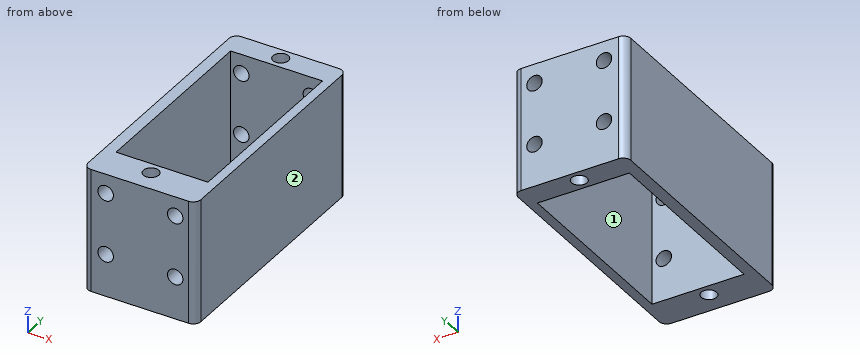
from build123d import *

# Parameters (mm, degrees)
SKETCH2_W           = 14.6
SKETCH2_H           = 32
BOSS_EXTRUDE1_DEPTH = 16
FILLET1_R           = 1
SKETCH3_W           = 11.9
SKETCH3_H           = 24.4
CUT_EXTRUDE1_DEPTH  = 16
SKETCH4_R           = 1
CUT_EXTRUDE2_DEPTH  = 16
SKETCH5_R           = 1
CUT_EXTRUDE3_DEPTH  = 113.555199241


with BuildPart() as part:
    # Sketch2 → Boss-Extrude1 (new body)
    with BuildSketch(Plane.XY):
        with Locations((-99.41772522, 219.327818509)):
            Rectangle(SKETCH2_W, SKETCH2_H)
    extrude(amount=BOSS_EXTRUDE1_DEPTH)

    # Fillet1
    fillet1_edges = [part.edges().sort_by_distance(p)[0] for p in [
        (-106.71772522, 235.327818509, 8),
        (-92.11772522, 235.327818509, 8),
        (-92.11772522, 203.327818509, 8),
        (-106.71772522, 203.327818509, 8),
    ]]
    fillet(fillet1_edges, radius=FILLET1_R)

    # Sketch3 → Cut-Extrude1 (cut)
    with BuildSketch(Plane.XY.offset(16)):
        with Locations((-99.26772522, 219.999996948)):
            Rectangle(SKETCH3_W, SKETCH3_H)
    extrude(amount=-CUT_EXTRUDE1_DEPTH, mode=Mode.SUBTRACT)

    # Sketch4 → Cut-Extrude2 (cut)
    with BuildSketch(Plane.XY.offset(16)):
        with Locations((-99.709122305, 233.799996948)):
            Circle(SKETCH4_R)
        with Locations((-99.709122305, 206.199996948)):
            Circle(SKETCH4_R)
    extrude(amount=-CUT_EXTRUDE2_DEPTH, mode=Mode.SUBTRACT)

    # Sketch5 → Cut-Extrude3 (cut, through all)
    with BuildSketch(Plane(origin=(0, 235.327818509, 0), x_dir=(1, 0, 0), z_dir=(0, 1, 0))):
        with Locations(Location((-103.837557169, -5.5, 0), (0, 0, 270))):
            Circle(SKETCH5_R)
        with Locations(Location((-94.837557169, -5.5, 0), (0, 0, 270))):
            Circle(SKETCH5_R)
        with Locations(Location((-94.837557169, -13.5, 0), (0, 0, 270))):
            Circle(SKETCH5_R)
        with Locations(Location((-103.837557169, -13.5, 0), (0, 0, 270))):
            Circle(SKETCH5_R)
    extrude(amount=-CUT_EXTRUDE3_DEPTH, mode=Mode.SUBTRACT)


solid = part.part
Can you work these out from the model? Positions are in its coordinate system, mm. Face numbers are marked on the shaded views. A direction names the side the tool comes from. Coordinates: 2 decimals unless noted, no trailing zeros. Loops run counter-clockwise (first coordinate to the right, second up) from the corner with the lowest first, then second, coordinate; pieces in that order, holes last. Notation, with made-up numbers: (37.25, 0) - (95.25, 0) arc R31 ccw to (95.25, 35) - close; hole circle Ø5 at (52.25, -1). An arc over 180 degrees is marked (long way). Answer as a JSON object with one key per item and string values. Group by question number.
Item 1: If we section it at A-A (z = 13.5): State how many separate pieces and enclosed holes the cut face has, plus the area to 3 significant figures.
Item 2: On a 3-axis mill with a long thin cutter (end or side, diameter ignored), from which of +Z, -Z, +X, -X, +Y, -Y can I reach the whole of each face in a straight line? I mean the marked faces 1 and 2. Say none if no direction works.
Item 3: If I drill on L1, parallel to X at y = 204.2, z = 5.5; L2, parallel to Y at x = -98.5, z = 8; L3, parallel to X at y = 230.5, z = 14, over which ranges is the centre line in solid material (lowest first)? Write a range as from..to.
Item 4: If we section it at C-C (y = 210.5): List the corners of the cut face in (x, z) for me, plus the area to 3 significant figures.
Item 5: If we section it at B-B (z = 11): List the corners of the cut face in (x, y) for me.
Item 6: If we section it at D-D (x = -99.25): List the corners of the cut face in (y, z) for me, plus the area to 3 significant figures.
Returned:
{
 "1": {"separate pieces": "4", "enclosed holes": "2", "area": "139 mm²"},
 "2": {"face 1": "+Z, -Z", "face 2": "+Z, -Z, +X, +Y, -Y"},
 "3": {"L1": "x = -106.71..-104.84, -102.84..-95.84, -93.84..-92.13", "L2": "y = 203.33..207.8, 232.2..235.33", "L3": "x = -106.72..-105.22, -93.32..-92.12"},
 "4": {"outline": "(-106.72, 0) - (-105.22, 0) - (-105.22, 16) - (-106.72, 16) - close; (-93.32, 0) - (-92.12, 0) - (-92.12, 16) - (-93.32, 16) - close", "area": "43.2 mm²"},
 "5": {"outline": "(-106.72, 204.33) arc R1 ccw to (-105.72, 203.33) - (-93.12, 203.33) arc R1 ccw to (-92.12, 204.33) - (-92.12, 234.33) arc R1 ccw to (-93.12, 235.33) - (-105.72, 235.33) arc R1 ccw to (-106.72, 234.33) - close; hole (-105.22, 207.8) - (-93.32, 207.8) - (-93.32, 232.2) - (-105.22, 232.2) - close; hole circle Ø2 at (-99.71, 206.2); hole circle Ø2 at (-99.71, 233.8)"},
 "6": {"outline": "(203.33, 0) - (205.31, 0) - (205.31, 16) - (203.33, 16) - close; (207.09, 0) - (207.8, 0) - (207.8, 16) - (207.09, 16) - close; (232.2, 0) - (232.91, 0) - (232.91, 16) - (232.2, 16) - close; (234.69, 0) - (235.33, 0) - (235.33, 16) - (234.69, 16) - close", "area": "64.7 mm²"}
}
